Autodesk Inventor part; units mm, degrees
ref_plane "Work Plane1" through (30, 0, 0) normal (0, -0.5, 0.866) x (1, 0, 0)
ref_plane "YZ Plane" through (0, 0, 0) normal (1, 0, 0) x (0, 1, 0)
ref_plane "XZ Plane" through (0, 0, 0) normal (0, 1, 0) x (-1, 0, 0)
sketch "Sketch1" plane through (0, 0, 0) normal (0, 0, 1) x (1, 0, 0)
  line L0 (-0.0667, 0) -> (16, 0)
  line L1 (16, 0) -> (16, 2)
  line L2 (16, 2) -> (1.4, 2)
  line L3 (1.4, 2) -> (0.9706, 2)
  line L4 (0.9706, 2) -> (0, 2)
  line L5 (0, 2) -> (0, 3.8)
  line L6 (0, 3.8) -> (-2.2, 3.8)
  line L7 (-2.2, 3.8) -> (-2.2, 1.4434)
  line L8 (-2.2, 1.4434) -> (-0.9, 1.4434)
  line L9 (-0.9, 1.4434) -> (-0.0667, 0)
  line L10 (-5.84, 0) -> (19.64, 0)
  line L11 (0, -0.76) -> (0, 4.56)
  line L12 (1.4, 2) -> (0, 2) construction
  dimension "d0" = 14.6
  dimension "d1" = 0.4294
  dimension "d2" = 2.2
  dimension "d3" = 1.3
  dimension "d4" = 60
  dimension "d5" = 4
  dimension "d6" = 4
  dimension "d7" = 2.8868
  dimension "d8" = 7.6
  dimension "d19" = 16
revolve "Body" add sketch "Sketch1" angle 360 about axis through (-0.0667, 0, 0) along (1, 0, 0)
sketch "Sketch2" plane through (-2.2, 0, 0) normal (-1, 0, 0) x (0, 0, 1)
  circle A0 centre (0, 0) radius 1.4434
  line L0 (0, -5.32) -> (0, 5.32)
  line L1 (-5.32, 0) -> (5.32, 0)
  line L2 (1.4434, 0) -> (0.7217, -1.25)
  line L3 (0.7217, -1.25) -> (-0.7217, -1.25)
  line L4 (-0.7217, -1.25) -> (-1.4434, 0)
  line L5 (-1.4434, 0) -> (-0.7217, 1.25)
  line L6 (-0.7217, 1.25) -> (0.7217, 1.25)
  line L7 (0.7217, 1.25) -> (1.4434, 0)
  point P0 (0, 0)
extrude "Slot" add sketch "Sketch2" against normal up to next contours L7 A0 | A0 L2 | L6 L0 A0 | A0 L0 L3 | L0 L6 A0 | A0 L3 L0 | L4 A0 | A0 L5
fillet "Fillet1" radius 1.82 1 edges at (-2.2, -3.8, 0)
thread "Thread"
chamfer "Chamfer1" distance 0.4294 distance2 0.4294 1 edges at (16, -2, 0) measured on face at (16, 0.527, -0.2661)
fillet "Fillet2" radius 0.2 1 edges at (0, -2, 0)
ref_plane "Work Plane1" through (30, 0, 0) normal (0, -0.5, 0.866) x (1, 0, 0)
equation "\"d0\" = GEL"
equation "\"d1\" = GAL"
equation "\"d2\" = KOH"
equation "\"d3\" = INTI"
equation "\"d5\" = GD"
equation "\"d6\" = BDM"
equation "\"d7\" = 1.1547 * SW"
equation "\"d8\" = KOD"
equation "\"d19\" = NLG"
equation "\"d16\" = RR"
equation "\"d12\" = GEL"
equation "\"d14\" = -0.5 * SPD + 0.5 * GD"
equation "\"d15\" = GUL"
equation "\"d29\" = R"
equation "\"GD\" = NND"
equation "\"NLG\" = 16"
equation "\"GEL\" = 14.6"
equation "\"KOD\" = 7.6"
equation "\"KOH\" = 2.2"
equation "\"INTI\" = 1.3"
equation "\"GAL\" = 0.61345 * PTC"
equation "\"GUL\" = 0.61345 * PTC"
equation "\"BDM\" = NND"
equation "\"SW\" = 2.5"
equation "\"RR\" = 1.82"
equation "\"SPD\" = 3.14117"
equation "\"d28\" = R"
equation "\"R\" = 0.2"
equation "\"TOA\" = 30deg"
equation "\"THREADDIA\" = 4"
equation "\"KOD1\" = KOD - 2 * RR"
equation "\"PTC\" = 0.7"
equation "\"NND\" = 4"
equation "\"E0\" = 1.155 * SW"
equation "\"GD1\" = THREADDIA - 1.2269 * PTC"
properties part number "11-4116" material "Steel, Mild"
Source: CAD feature listing. Evaluate the final solid. Frame: model axes, mm. A direction names the side the tool comes from. Give positions to 0.01 mm unless a question says otherwise; leave off trailing zeros. Write each loop counter-clockwise with the first axis right and the second up, starting at its lowest first coordinate (ties: lowest second). Pieces come first, ordered by that corner, then holes.
1. Material intervals for line 1 along Z through (x, y) = (12.5, 0.25); line 2 along Y through (x, z) = (12, -0.75); line 3 along X through (y, z) = (0, -0.5), sorted ascending.
2. Section query A-A (x = 5.75). Return the cut outline in (y, z).
3. Access query for faces 4 (the face through (16, 0, 0)), 5 (the face through (-1.5, -0.63, -1.08)). Directions: +Z, -Z, +X, -X, +Y, -Y. A direction counts if a zero-diameter tool reaches every point of the face in a straight line with its end or side. Return the directions, or none.
4. Pull-direction query (Z, two-part tool) for faces 1 (the face through (0, 2, -2)), 2 (the face through (8, 0, 2)), 3 (the face through (-1.504, -0.616, 1.088)); classes: +Z half, -Z half, draft (parallel to the pull), parting line (faces both ways), or undercut.
5. First-contact query: pin 1 (4 mm diameter, centred on y = 2, z = -1, fed in from -X); pin 2 (4 mm diameter, centred on x = 3, y = 2, fed in from -Z); pin 3 (1.6 mm diameter, centred on x = -1.5, z = 0, fed in from +Y); pin 4 (1 mm diameter, centred on x = 4.5, z = 1.5, fed in from -Y). Flat tips, straight axial feed; report the tip coordinate or a pass-through.
Output values:
1. line 1: z = -1.98 to 1.98
1. line 2: y = -1.85 to 1.85
1. line 3: x = -0.36 to 16
2. outline: circle Ø4 at (0, 0)
3. face 4: +Z, -Z, +X, +Y, -Y
3. face 5: -X
4. face 1: draft
4. face 2: parting line
4. face 3: undercut
5. pin 1: stops at x = -2.2
5. pin 2: stops at z = -2
5. pin 3: stops at y = 3.77
5. pin 4: stops at y = -1.73
